```python
from build123d import *

# Parameters (mm, degrees)
F1_DEPTH       = 9.652
F3_D           = 5.461
F3_CBORE_D     = 9.779
F3_CBORE_DEPTH = 5.588
F5_D           = 19.05
F7_D           = 4.2
F7_DEPTH       = 12.7
F7_TIP         = 1.2618073
F9_D           = 4.2
F9_DEPTH       = 12.7
F9_TIP         = 1.2618073
F11_D          = 4.2
F11_DEPTH      = 17.272
F11_TIP        = 1.2618073


with BuildPart() as f1:
    # F0 (on Front) → F1 (new body)
    with BuildSketch(Plane.XZ):
        Polygon((-79.8280344415, 30.48), (-79.8280344415, 0), (113.9739655585, 0), (113.9739655585, 68.072), (85.9069655585, 68.072), (85.9069655585, 30.48), align=None)
    extrude(amount=-F1_DEPTH)

    # F3 (through all)
    with Locations(Plane.XZ):
        with Locations((73.2069655585, 15.24), (101.1469655585, 15.24)):
            CounterBoreHole(F3_D / 2, F3_CBORE_D / 2, F3_CBORE_DEPTH)

    # F5 (through all)
    with Locations(Plane.XZ):
        with Locations((99.8769655585, 54.102)):
            Hole(F5_D / 2)

    # F7
    with Locations(Plane.XY.offset(68.072)):
        with Locations((99.9404655585, 4.826)):
            Hole(F7_D / 2, depth=F7_DEPTH)
            with Locations((0, 0, -(F7_DEPTH + F7_TIP / 2))):  # 118° drill point
                Cone(0, F7_D / 2, F7_TIP, mode=Mode.SUBTRACT)

    # F9
    with Locations(Plane.YZ.offset(113.9739655585)):
        with Locations((4.826, 54.063147307)):
            Hole(F9_D / 2, depth=F9_DEPTH)
            with Locations((0, 0, -(F9_DEPTH + F9_TIP / 2))):  # 118° drill point
                Cone(0, F9_D / 2, F9_TIP, mode=Mode.SUBTRACT)

    # F11
    with Locations(Plane(origin=(-79.8280344415, 0, 0), x_dir=(0, -1, 0), z_dir=(-1, 0, 0))):
        with Locations((-4.826, 20.32), (-4.826, 10.16)):
            Hole(F11_D / 2, depth=F11_DEPTH)
            with Locations((0, 0, -(F11_DEPTH + F11_TIP / 2))):  # 118° drill point
                Cone(0, F11_D / 2, F11_TIP, mode=Mode.SUBTRACT)


with BuildPart() as f12_1:
    # F12: copy of F1
    add(f1.part)


solid = f1.part
```
The model under review builds one solid part; all positions refer to its coordinate system, in mm. A direction names the side the tool comes from. Give positions to 0.01 mm unless a question says otherwise; leave off trailing zeros. Write each loop counter-clockwise with the first axis right and the second up, starting at its lowest first coordinate (ties: lowest second). Pieces come first, ordered by that corner, then holes. Notation, with made-up numbers: M -27,16.25 L -19,16.25 A27 cw -19,51.25 Z; hole C 29,-8.5 d7. An arc over 180 degrees is marked long. Write each question's results on one line, items separated by ' | '. Start each with the question number.
1. For faces 5 (the cylindrical face through (98, 4.02, 65.69)), 6 (the flat face through (103, 5.588, 13)), 7 (the cylindrical face through (-71.07, 4.37, 8.11)), 8 (the flat face through (4, 5, 30.48)), list the 3-axis set-ups (+Z, -Z, +X, -X, +Y, -Y) from which the entire face can be reached by the end or side of a thin tool; tool diameter is ignored.
2. For probe 1 along X at (y, z) = (4.5, 19.5); probe 2 along Y at (x, z) = (-75, 10.16); probe 3 along Y at (x, z) = (104, 18.5), list the stretches that pass through material, from the lowest coordinate up. Write a range as [from, to].
3. Mouldability with a two-part tool opening along Z and no side actions: class faces 1 (the cylindrical face through (111.53, 2.82, 54.69)), 2 (the flat face through (75.3, 5.588, 13.1)), 3 (the flat face through (103, 5, 68.072)), 4 (the flat face through (113.974, 5, 34)) as released by +Z, released by -Z, zero draft, split by the parting line, or undercut.
4. We need section A-A (z = 15.24). Write out the cut boundary in (x, y).
5. We need section C-C (z = 33). Write out the cut boundary in (x, y), and give its area (3 significant figures).
6. Insertion check: pin 1 Ø4 at (x, y) = (99.94, 4.83) entering from +Z; pin 2 Ø1.5 at (x, y) = (40, 7.5) entering from +Z; pin 3 Ø3.5 at (y, z) = (4.826, 20.32) entering from -X. Each pin has a flat end and moves straight along its axis. Give the tip position at first contact, or say it passes through.
7. We need section B-B (x = -18). Write out the cut boundary in (y, z), and give its area (3 significant figures).
Results found:
1) face 5: +Z | face 6: -Y | face 7: -X | face 8: +Z, -X, +Y, -Y
2) probe 1: x = [-61.82, 70.81], [75.61, 98.75], [103.55, 113.97] | probe 2: y = [0, 2.73], [6.93, 9.65] | probe 3: y = [5.59, 9.65]
3) face 1: undercut | face 2: undercut | face 3: released by +Z | face 4: zero draft
4) outline: M -79.83,0 L 68.32,0 L 68.32,5.59 L 70.48,5.59 L 70.48,9.65 L -79.83,9.65 Z; M 75.94,5.59 L 78.1,5.59 L 78.1,0 L 96.26,0 L 96.26,5.59 L 98.42,5.59 L 98.42,9.65 L 75.94,9.65 Z; M 103.88,5.59 L 106.04,5.59 L 106.04,0 L 113.97,0 L 113.97,9.65 L 103.88,9.65 Z
5) outline: M 85.91,0 L 113.97,0 L 113.97,9.65 L 85.91,9.65 Z | area: 271 mm^2
6) pin 1: stops at z = 44.8 | pin 2: stops at z = 30.48 | pin 3: stops at x = -62.35
7) outline: M 0,0 L 9.65,0 L 9.65,30.48 L 0,30.48 Z | area: 294 mm^2
